from build123d import *

# Parameters (mm, degrees)
SKETCH2_R               = 50
BOSS_EXTRUDE1_DEPTH     = 12
SKETCH3_R               = 48
CUT_EXTRUDE1_DEPTH      = 10
SKETCH7_W               = 10
SKETCH7_H               = 10
BOSS_EXTRUDE12_DEPTH    = 3
SKETCH8_W               = 10
SKETCH8_H               = 10
BOSS_EXTRUDE13_DEPTH    = 3
SKETCH9_R               = 3.5
CUT_EXTRUDE2_DEPTH      = 10
SKETCH10_R              = 3.5
CUT_EXTRUDE3_DEPTH      = 10
CUT_EXTRUDE4_DEPTH      = 100
CUT_EXTRUDE4_DEPTH_BACK = 100
SKETCH11_W              = 125.880590586
SKETCH11_H              = 15.914036276
BOSS_EXTRUDE15_START    = -3
SKETCH12_R              = 48
BOSS_EXTRUDE15_DEPTH    = 3


with BuildPart() as part:
    # Sketch2 → Boss-Extrude1 (new body)
    with BuildSketch(Plane(origin=(0, 0, 0), x_dir=(1, 0, 0), z_dir=(0, 1, 0))):
        with Locations(Location((0, 0, 0), (0, 0, 270))):
            Circle(SKETCH2_R)
    extrude(amount=BOSS_EXTRUDE1_DEPTH)

    # Sketch3 → Cut-Extrude1 (cut)
    with BuildSketch(Plane.XZ):
        with Locations(Location((0, 0, 0), (0, 0, 270))):
            Circle(SKETCH3_R)
    extrude(amount=-CUT_EXTRUDE1_DEPTH, mode=Mode.SUBTRACT)

    # Sketch7 → Boss-Extrude12 (add)
    with BuildSketch(Plane(origin=(0, 0, 0), x_dir=(-1, 0, 0), z_dir=(0, -1, 0))):
        with Locations((0, 54.749371855)):
            Rectangle(SKETCH7_W, SKETCH7_H)
    extrude(amount=-BOSS_EXTRUDE12_DEPTH)

    # Sketch8 → Boss-Extrude13 (add)
    with BuildSketch(Plane(origin=(0, 0, 0), x_dir=(-1, 0, 0), z_dir=(0, -1, 0))):
        with Locations((0, -54.749371855)):
            Rectangle(SKETCH8_W, SKETCH8_H)
    extrude(amount=-BOSS_EXTRUDE13_DEPTH)

    # Sketch9 → Cut-Extrude2 (cut)
    with BuildSketch(Plane.XZ):
        with Locations(Location((0, 54.549371855, 0), (0, 0, 270))):
            Circle(SKETCH9_R)
    extrude(amount=-CUT_EXTRUDE2_DEPTH, mode=Mode.SUBTRACT)

    # Sketch10 → Cut-Extrude3 (cut)
    with BuildSketch(Plane.XZ):
        with Locations(Location((0, -54.549371855, 0), (0, 0, 270))):
            Circle(SKETCH10_R)
    extrude(amount=-CUT_EXTRUDE3_DEPTH, mode=Mode.SUBTRACT)

    # Sketch11 → Cut-Extrude4 (cut, two sides: drawn at the far end of the back side and taken through both)
    with BuildSketch(Plane(origin=(5, 0, 0), x_dir=(0, 0, -1), z_dir=(1, 0, 0)).offset(-CUT_EXTRUDE4_DEPTH_BACK)):
        with Locations((3.190923438, 10.957018138)):
            Rectangle(SKETCH11_W, SKETCH11_H)
    extrude(amount=CUT_EXTRUDE4_DEPTH + CUT_EXTRUDE4_DEPTH_BACK, mode=Mode.SUBTRACT)

    # Sketch12 → Boss-Extrude15 (add)
    with BuildSketch(Plane(origin=(0, 3, 0), x_dir=(1, 0, 0), z_dir=(0, 1, 0)).offset(BOSS_EXTRUDE15_START)):
        Circle(SKETCH12_R)
    extrude(amount=BOSS_EXTRUDE15_DEPTH)


solid = part.part
Read the model definition and answer for the solid it produces. Units are mm, in the model's axes. A direction names the side the tool comes from. Give positions to 0.01 mm unless a question says otherwise; leave off trailing zeros. Write each loop counter-clockwise with the first axis right and the second up, starting at its lowest first coordinate (ties: lowest second). Pieces come first, ordered by that corner, then holes. Notation, with made-up numbers: (-21, 26.5) - (-11, 26.5) arc R20 cw to (-11, 36.5) - close; hole circle Ø9 at (68.5, -1.5). An arc over 180 degrees is marked (long way). Answer in a Markdown table with one row per item. Add a question column.
Item 1: Determine the mould class of faces 6 (the face through (-1, 0, -1)), 7 (the face through (1.05, 1.48, -57.89)), 8 (the face through (49.99, 1.48, 1.03)), 9 (the face through (-5, 1, -55)) for opening direction X: pulls with the +X half, pulls with the -X half, needs draft (parallel to the pull), parting line crosses it, or undercut.
Item 2: Section D-D, the plane z = -18 is taken. Write down the section's boundary in (x, y), and give its area (3 significant figures).
Item 3: Flat-ended cylindrical pins translate along their axes: P1, Ø0.9, axis at y = 1.5, z = -52.5, coming from the -X side; P2, Ø1.5, axis at x = 20.5, y = 0.5, coming from the +Z side; P3, Ø4, axis at x = 0, z = -54.55, coming from the -Y side; P4, Ø1.5, axis at y = 2, z = -53.5, coming from the +X side. Find the tip coordinate at first contact, or state that the pin passes through.
Item 4: Section C-C, the plane z = 52.5 is taken. Write down the section's boundary in (x, y).
Item 5: Section B-B, the plane y = 2.15 is taken. Write down the section's boundary in (x, z), and give its area (3 significant figures).
Item 6: Find the intervals of material crossed by L1, parallel to Z at x = 2.5, y = 2; L2, parallel to X at y = 1, z = 52.5; L3, parallel to Z at x = -2, y = 1.25, in increasing order.
Item 7: A tool of negligible diameter and unlimited length cuts with its end or side. For faces 1 (the face through (0, 1, 59.749)), 2 (the face through (5, 1, 55)), 3 (the face through (-5, 1, 55)), 4 (the face through (-49.99, 1.48, -1.03)), 5 (the face through (5, 1, -55)), from which of +Z, -Z, +X, -X, +Y, -Y can it reach the whole face along a straight path? Write none if from no direction.
Item 8: Section A-A, the plane x = 0 is taken. Write down the section's boundary in (y, z), and give its area (3 significant figures).
Recorded:
| question | item | result |
|---|---|---|
| 1 | face 6 | needs draft |
| 1 | face 7 | undercut |
| 1 | face 8 | pulls with the +X half |
| 1 | face 9 | pulls with the -X half |
| 2 | outline | (-46.65, 0) - (46.65, 0) - (46.65, 3) - (-46.65, 3) - close |
| 2 | area | 280 mm2 |
| 3 | P1 | stops at x = -5 |
| 3 | P2 | stops at z = 45.93 |
| 3 | P3 | passes through |
| 3 | P4 | stops at x = 5 |
| 4 | outline | (-5, 0) - (-2.84, 0) - (-2.84, 3) - (-5, 3) - close; (2.84, 0) - (5, 0) - (5, 3) - (2.84, 3) - close |
| 5 | outline | (-5, -59.75) - (5, -59.75) - (5, -49.75) arc R50 ccw to (5, 49.75) - (5, 59.75) - (-5, 59.75) - (-5, 49.75) arc R50 ccw to (-5, -49.75) - close; hole circle Ø7 at (0, -54.55); hole circle Ø7 at (0, 54.55) |
| 5 | area | 7,970 mm2 |
| 6 | L1 | z = -59.75 to -57, -52.1 to 52.1, 57 to 59.75 |
| 6 | L2 | x = -5 to -2.84, 2.84 to 5 |
| 6 | L3 | z = -59.75 to -57.42, -51.68 to 51.68, 57.42 to 59.75 |
| 7 | face 1 | +Z, +X, -X, +Y, -Y |
| 7 | face 2 | +Z, +X, +Y, -Y |
| 7 | face 3 | +Z, -X, +Y, -Y |
| 7 | face 4 | -X, +Y, -Y |
| 7 | face 5 | -Z, +X, +Y, -Y |
| 8 | outline | (0, -59.75) - (3, -59.75) - (3, -58.05) - (0, -58.05) - close; (0, -51.05) - (3, -51.05) - (3, 51.05) - (0, 51.05) - close; (0, 58.05) - (3, 58.05) - (3, 59.75) - (0, 59.75) - close |
| 8 | area | 316 mm2 |
